```python
from build123d import *

# Parameters (mm, degrees)
F0_R     = 3.625
F1_DEPTH = 2.75
F3_DEPTH = 1.5
F4_R     = 3.5
F5_DEPTH = 0.5
F7_R     = 0.1


# Not quite as in the source:
# - a fillet or chamfer that OpenCascade refuses, or shapes differently, is made with other operations: its cross-section is extruded or revolved along the edge and cut away or added


with BuildPart() as f1:
    # F0 (on Right) → F1 (new body, symmetric)
    with BuildSketch(Plane.YZ):
        Circle(F0_R)
    extrude(amount=F1_DEPTH, both=True)

    # F2 (on face) → F3 (join)
    with BuildSketch(Plane(origin=(-2.75, 0, 0), x_dir=(0, -1, 0), z_dir=(-1, 0, 0))):
        with BuildLine():
            Line((3.5465652398, -0.75), (5.0465652398, -0.75))
            Line((5.0465652398, -0.75), (5.0465652398, 0.75))
            Line((5.0465652398, 0.75), (3.5465652398, 0.75))
            ThreePointArc((3.5465652398, 0.75), (3.625, 0), (3.5465652398, -0.75))
        make_face()
        with BuildLine():
            Line((-3.5465652398, 0.75), (-5.0465652398, 0.75))
            Line((-5.0465652398, 0.75), (-5.0465652398, -0.75))
            Line((-5.0465652398, -0.75), (-3.5465652398, -0.75))
            ThreePointArc((-3.5465652398, -0.75), (-3.625, 0), (-3.5465652398, 0.75))
        make_face()
    extrude(amount=-F3_DEPTH)

    # F4 (on face) → F5 (cut)
    with BuildSketch(Plane.YZ.offset(2.75)):
        Circle(F4_R)
    extrude(amount=-F5_DEPTH, mode=Mode.SUBTRACT)

    # F6: fillet of radius 9 on 1 edges, made by hand

    # F6_s1 → F6_t2 (revolve)
    with BuildSketch(Plane.XY):
        with BuildLine():
            ThreePointArc((2.75, 3.5), (2.3758803254, 2.0419601084), (2.25, 0.5419601084))
            Line((2.25, 0.5419601084), (2.25, 3.5))
            Line((2.25, 3.5), (2.75, 3.5))
        make_face()
    revolve(axis=Axis((2.25, 0, 0), (1, 0, 0)))

    # F7
    f7_edges = [f1.edges().sort_by_distance(p)[0] for p in [
        (2.75, -3.5, 0),
        (2.75, -3.625, 0),
    ]]
    fillet(f7_edges, radius=F7_R)


solid = f1.part
```
Input: part model. Units: mm. Frame: model coordinates. A direction names the side the tool comes from. Coordinates: 2 decimals unless noted, no trailing zeros. Write each loop counter-clockwise with the first axis right and the second up, starting at its lowest first coordinate (ties: lowest second). Pieces come first, ordered by that corner, then holes. Notation, with made-up numbers: (26.25, 21) - (57.25, 21) arc R22 cw to (57.25, 31) - close; hole circle Ø1 at (-12, 14.5). An arc over 180 degrees is marked (long way). Put each result on its own line as item: value. Start each with the question number.
1) Reachability of faces 1 (the face through (-2, 4, -0.75)), 2 (the face through (-2, -4, -0.75)), 3 (the face through (-2, -4, 0.75)) from +Z, -Z, +X, -X, +Y, -Y: full face, straight path, thin tool, end or side. Return the list, or none.
2) Contact query for flat-ended pins moving along their axis: pin 1 (1.6 mm diameter, centred on x = -2, y = 4.5, fed in from +Z); pin 2 (2 mm diameter, centred on x = -1, z = 3, fed in from +Y); pin 3 (0.8 mm diameter, centred on y = -4.5, z = 0, fed in from +X). Output: stop coordinate, or through.
3) Cut plane A-A (x = 2). Return the cut outline in (y, z) (3 decimals).
4) Cut plane B-B (y = -4.5). Return the cut outline in (x, z), plus the area to 3 significant figures.
5) Mould query, pull axis Y, two halves, no side actions, for faces 4 (the face through (-0.012, 3.458, 1.089)), 5 (the face through (-2, 4, 0.75)), 6 (the face through (-2, -5.047, 0)), 7 (the face through (2.25, 0, 0)). Classes: pulls with the +Y half, pulls with the -Y half, needs draft (parallel to the pull), parting line crosses it, or undercut.
6) Ray query, L1, parallel to X at y = 0.75, z = -0.25; L2, parallel to Z at x = 1.85, y = -1; L3, parallel to Y at x = 2.2, z = 0 (3 decimals). Return the intervals inside material, ascending.
Resolved:
1. face 1: -Z, +X, -X, +Y
1. face 2: -Z, +X, -X, -Y
1. face 3: +Z, +X, -X, -Y
2. pin 1: stops at z = 0.75
2. pin 2: stops at y = 3.02
2. pin 3: stops at x = -1.25
3. outline: circle Ø7.25 at (0, 0)
4. outline: (-2.75, -0.75) - (-1.25, -0.75) - (-1.25, 0.75) - (-2.75, 0.75) - close
4. area: 2.25 mm2
5. face 4: parting line crosses it
5. face 5: needs draft
5. face 6: pulls with the -Y half
5. face 7: undercut
6. L1: x = -2.75 to 2.25
6. L2: z = -3.48 to 3.48
6. L3: y = -3.625 to 3.625
